Can you work these out from the drawing? Everything is in mm from the part's minimum corner. Round coordinates to 2 decimals unless told otherwise and drop trailing zeros. Loops run counter-clockwise (first coordinate to the right, second up) from the corner with the lowest first, then second, coordinate; pieces in that order, holes last. Notation, with made-up numbers: M 65.25,-14.5 L 69.25,-14.5 A34 ccw 69.25,21.5 Z; hole C -30,15 d9. An arc over 180 degrees is marked long. Use a Markdown table: item, result.
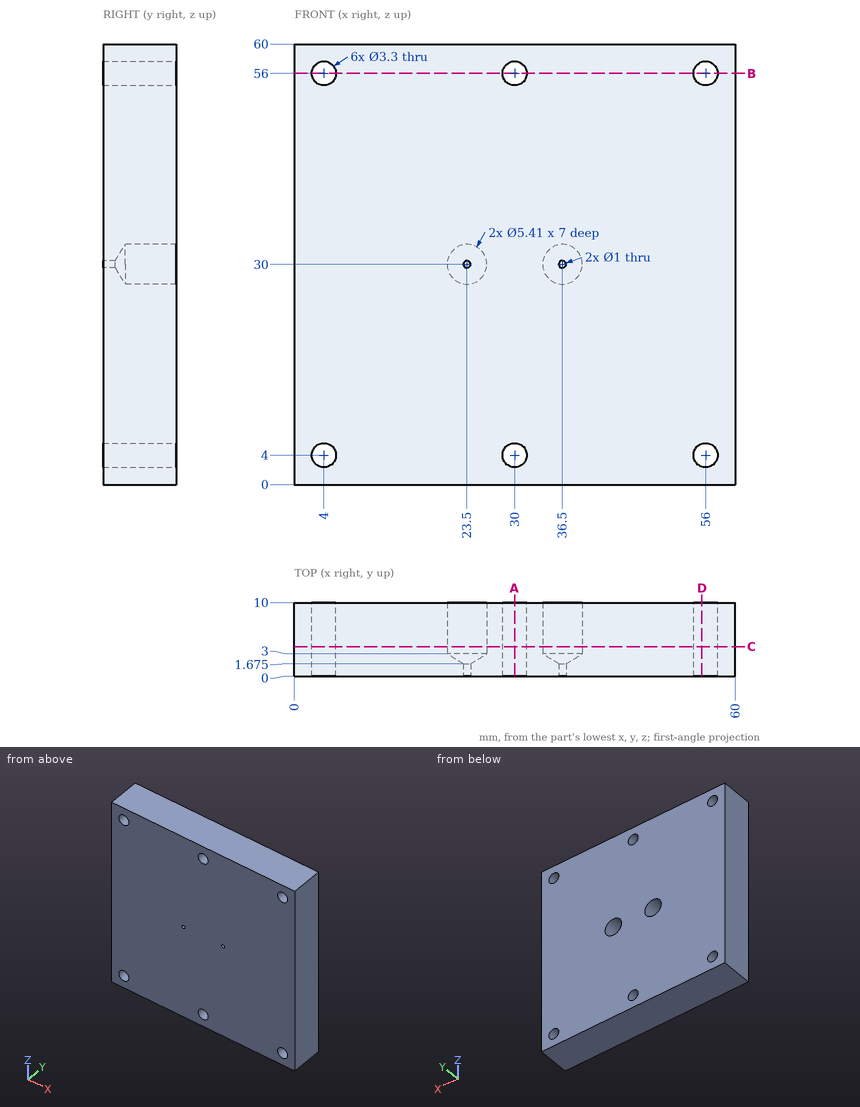
1. Imagine slicing it at A-A, the plane x = 30. Write out the boundary of the cut face in (y, z).
Answer sheet:
| item | result |
|---|---|
| outline | M 0,0 L 10,0 L 10,2.35 L 0,2.35 Z; M 0,5.65 L 10,5.65 L 10,54.35 L 0,54.35 Z; M 0,57.65 L 10,57.65 L 10,60 L 0,60 Z |
2. Imagine slicing it at B-B, the plane z = 56. Write out the boundary of the cut face in (x, y), then the cut area to 3 significant figures.
Answer sheet:
| item | result |
|---|---|
| outline | M 0,0 L 2.35,0 L 2.35,10 L 0,10 Z; M 5.65,0 L 28.35,0 L 28.35,10 L 5.65,10 Z; M 31.65,0 L 54.35,0 L 54.35,10 L 31.65,10 Z; M 57.65,0 L 60,0 L 60,10 L 57.65,10 Z |
| area | 501 mm2 |
3. Imagine slicing it at C-C, the plane y = 4. State how many separate pieces and enclosed holes the cut face has, then the cut area to 3 significant figures.
Answer sheet:
| item | result |
|---|---|
| separate pieces | 1 |
| enclosed holes | 8 |
| area | 3,500 mm2 |
4. For pin 1 Ø2 at (x, z) = (56, 56) entering from -Y; pin 2 Ø3 at (x, z) = (23.5, 30) entering from +Y, each with a flat end and sliding along its axis, tell me the tip position at first contact or that it passes through.
Answer sheet:
| item | result |
|---|---|
| pin 1 | through |
| pin 2 | y = 2.28 |
5. Imagine slicing it at D-D, the plane x = 55.5. Write out the boundary of the cut face in (y, z), then the cut area to 3 significant figures.
Answer sheet:
| item | result |
|---|---|
| outline | M 0,0 L 10,0 L 10,2.43 L 0,2.43 Z; M 0,5.57 L 10,5.57 L 10,54.43 L 0,54.43 Z; M 0,57.57 L 10,57.57 L 10,60 L 0,60 Z |
| area | 537 mm2 |
6. I need wall thicknesses on probe 1 along X at (y, z) = (2.5, 4); probe 2 along Z at (x, y) = (56, 2.75); probe 3 along X at (y, z) = (1.15, 30). Which ranges of each line are inside material? Lowest first, please. Write a range as from..to.
Answer sheet:
| item | result |
|---|---|
| probe 1 | 0..2.35, 5.65..28.35, 31.65..54.35, 57.65..60 |
| probe 2 | 0..2.35, 5.65..54.35, 57.65..60 |
| probe 3 | 0..23, 24..36, 37..60 |
